The model under review builds one solid part; all positions refer to its coordinate system, in mm. Face numbers are marked on the shaded views. Coordinates: 2 decimals unless noted, no trailing zeros. Order: outer loops, then holes, each group sorted by start corner. A loop starts at its lowest first (then second) coordinate and runs counter-clockwise, first axis right, second up. Notation, with made-up numbers: (18.5, 81.5) -> (28.5, 81.5) arc R16 cw to (28.5, 107.5) -> close; hole circle Ø4 at (34, -6). An arc over 180 degrees is marked (long way). Use one line per item in the form item = value. Start each with the question number.
(1) Take a section at B-B (y = 4). State the section outline as (x, z) points, then the cut area to 3 significant figures.
(2) Wall thickness on line 1 along Z through (x, y) = (10, 8); line 2 along X through (y, z) = (1.4, -20.5); line 3 along Z through (x, y) = (16.5, 9.5): over which ranges is each line inside the solid? List them lowest first.
(3) Take a section at C-C (z = 18.5). State the section outline as (x, y) points, then the cut area to 3 significant figures.
(4) Insertion check: pin 1 Ø6.5 at (x, z) = (5, -7) entering from +Y; pin 2 Ø1 at (y, z) = (6, 11) entering from +X; pin 3 Ø2 at (y, z) = (1, 8) entering from +X. Each pin has a flat end and moves straight along its axis. Give the tip position at first contact, or say it passes through.
(5) Take a section at D-D (x = 6). State the section outline as (y, z) points.
(6) Mouldability with a two-part tool opening along X and no side actions: class the marked faces 1, 2, 3 and 4 as +X half, -X half, draft (parallel to the pull), parting line (faces both ways), or undercut.
(7) Take a section at A-A (x = 16). State the section outline as (y, z) points.
```python
from build123d import *

# Parameters (mm, degrees)
BOSS_EXTRUDE1_DEPTH = 2
SKETCH2_W           = 5
SKETCH2_H           = 5
SKETCH2_W_2         = 37
SKETCH2_H_2         = 22
BOSS_EXTRUDE3_DEPTH = 18
SKETCH3_R           = 1.25
CUT_EXTRUDE1_DEPTH  = 38.003378224
FILLET1_R           = 1


with BuildPart() as part:
    # Sketch1 → Boss-Extrude1 (new body)
    with BuildSketch(Plane(origin=(0, 0, 0), x_dir=(1, 0, 0), z_dir=(0, 1, 0))):
        Polygon((20.5, 25), (20.5, -1), (-17.5, -1), (-17.5, -12), (20.5, -12), (20.5, -25), (-20.5, -25), (-20.5, 25), align=None)
    extrude(amount=BOSS_EXTRUDE1_DEPTH)

    # Sketch2 → Boss-Extrude3 (add)
    with BuildSketch(Plane(origin=(0, 2, 0), x_dir=(1, 0, 0), z_dir=(0, 1, 0))):
        Polygon((20.5, 25), (-20.5, 25), (-20.5, -25), (20.5, -25), (20.5, -12), (-17.5, -12), (-18.5, -12), (-18.5, -1), (-17.5, -1), (20.5, -1), align=None)
        with Locations((16, -18.5)):
            Rectangle(SKETCH2_W, SKETCH2_H, mode=Mode.SUBTRACT)
        with Locations((0, 12)):
            Rectangle(SKETCH2_W_2, SKETCH2_H_2, mode=Mode.SUBTRACT)
    extrude(amount=BOSS_EXTRUDE3_DEPTH)

    # Sketch3 → Cut-Extrude1 (cut, through all)
    with BuildSketch(Plane(origin=(0, 2, 0), x_dir=(1, 0, 0), z_dir=(0, 1, 0))):
        with Locations(Location((16, 20.5, 0), (0, 0, 270))):
            Circle(SKETCH3_R)
        with Locations(Location((16, -18.5, 0), (0, 0, 270))):
            Circle(SKETCH3_R)
    extrude(amount=-CUT_EXTRUDE1_DEPTH, mode=Mode.SUBTRACT)

    # Fillet1
    fillet1_edges = [part.edges().sort_by_distance(p)[0] for p in [
        (20.5, 20, -12),
        (0, 20, -25),
        (-20.5, 20, 0),
        (0, 20, 25),
        (20.5, 20, 18.5),
    ]]
    fillet(fillet1_edges, radius=FILLET1_R)


solid = part.part
```
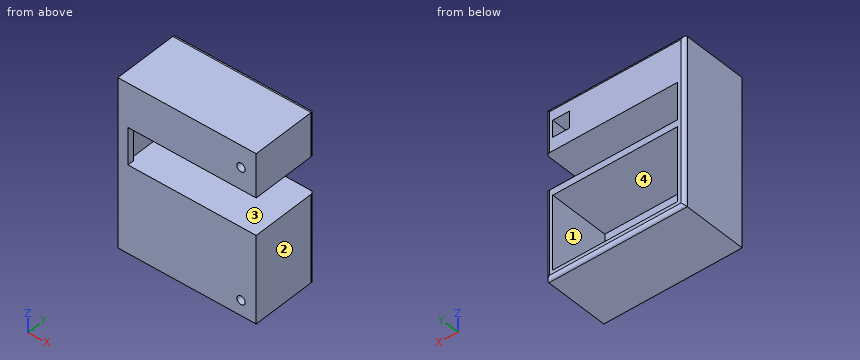
Findings:
q1.outline = (-20.5, -25) -> (20.5, -25) -> (20.5, 1) -> (-18.5, 1) -> (-18.5, 12) -> (20.5, 12) -> (20.5, 25) -> (-20.5, 25) -> close; hole (-18.5, -23) -> (18.5, -23) -> (18.5, -1) -> (-18.5, -1) -> close; hole (13.5, 16) -> (18.5, 16) -> (18.5, 21) -> (13.5, 21) -> close
q1.area = 782 mm²
q2.line_1 = -25 to -23, -1 to 1, 12 to 25
q2.line_2 = -20.5 to 14.75, 17.25 to 20.5
q2.line_3 = -25 to -23, -1 to 1, 12 to 16, 21 to 25
q3.outline = (-20.5, 0) -> (14.75, 0) -> (14.75, 2) -> (13.5, 2) -> (13.5, 20) -> (-19.5, 20) arc R1 ccw to (-20.5, 19) -> close; (17.25, 0) -> (20.5, 0) -> (20.5, 19) arc R1 ccw to (19.5, 20) -> (18.5, 20) -> (18.5, 2) -> (17.25, 2) -> close
q3.area = 725 mm²
q4.pin_1 = 2
q4.pin_2 = -18.5
q4.pin_3 = -17.5
q5.outline = (0, -25) -> (19, -25) arc R1 ccw to (20, -24) -> (20, -23) -> (2, -23) -> (2, -1) -> (20, -1) -> (20, 1) -> (0, 1) -> close; (0, 12) -> (20, 12) -> (20, 24) arc R1 ccw to (19, 25) -> (0, 25) -> close
q6.face_1 = undercut
q6.face_2 = +X half
q6.face_3 = draft
q6.face_4 = undercut
q7.outline = (0, -25) -> (19, -25) arc R1 ccw to (20, -24) -> (20, -23) -> (2, -23) -> (2, -21.75) -> (0, -21.75) -> close; (0, -19.25) -> (2, -19.25) -> (2, -1) -> (20, -1) -> (20, 1) -> (0, 1) -> close; (0, 12) -> (20, 12) -> (20, 16) -> (2, 16) -> (2, 17.25) -> (0, 17.25) -> close; (0, 19.75) -> (2, 19.75) -> (2, 21) -> (20, 21) -> (20, 24) arc R1 ccw to (19, 25) -> (0, 25) -> close
